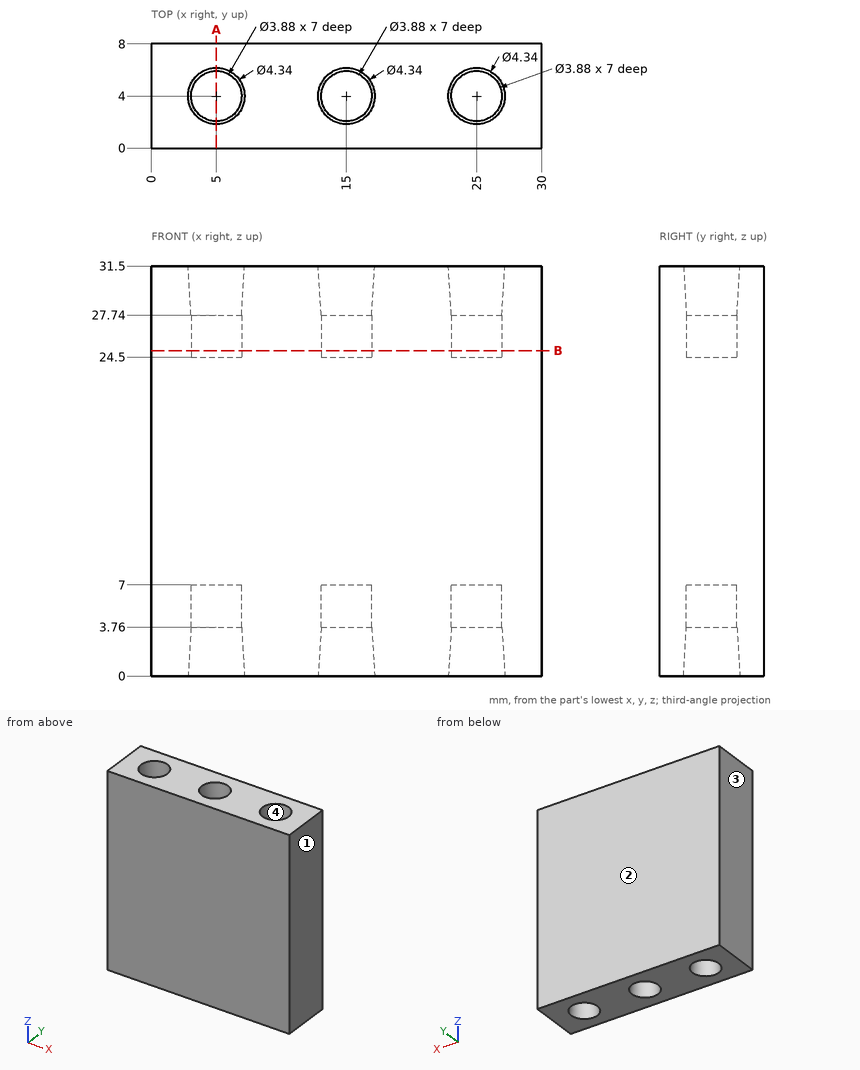
For this review, use the dimensioned drawing (mm, ordinates from the lowest corner) and the shaded views. Round coordinates to 2 decimals unless told otherwise and drop trailing zeros. Loops run counter-clockwise (first coordinate to the right, second up) from the corner with the lowest first, then second, coordinate; pieces in that order, holes last. Notation, with made-up numbers: M 14,43.5 L 58,43.5 A18 cw 58,68.5 Z; hole C -2,54 d2. An arc over 180 degrees is marked long. Answer as CSV lines item,"result".
1. Insertion check: pin 1 Ø3 at (x, y) = (15, 4) entering from +Z; pin 2 Ø1.2 at (x, y) = (4.5, 3) entering from -Z. Each pin has a flat end and moves straight along its axis. Give the tip position at first contact, or say it passes through.
Outcome:
pin 1,"stops at z = 24.5"
pin 2,"stops at z = 7"
2. To check wall thickness, follow L1, parallel to X at y = 4, z = 5.5; L2, parallel to Y at x = 25, z = 5.05; L3, parallel to Z at x = 26.25, y = 3.75. State the ranges of each line that lie inside material, in increasing order. Write a range as [from, to].
Outcome:
L1,"x = [0, 3.06], [6.94, 13.06], [16.94, 23.06], [26.94, 30]"
L2,"y = [0, 2.06], [5.94, 8]"
L3,"z = [7, 24.5]"
3. We need section B-B (z = 25). Give the boundary of the cut face in (x, y).
Outcome:
outline,"M 0,0 L 30,0 L 30,8 L 0,8 Z; hole C 5,4 d3.88; hole C 15,4 d3.88; hole C 25,4 d3.88"
4. Draft analysis for pull direction X (two halves, no side actions). For the marked faces 1, 2, 3 and 4, state which applies: pulls with the +X half, pulls with the -X half, needs draft (parallel to the pull), parting line crosses it, or undercut.
Outcome:
face 1,"pulls with the +X half"
face 2,"needs draft"
face 3,"pulls with the -X half"
face 4,"undercut"
5. We need section A-A (x = 5). Give the boundary of the cut face in (y, z).
Outcome:
outline,"M 0,0 L 1.83,0 L 2.06,3.76 L 2.06,7 L 5.94,7 L 5.94,3.76 L 6.17,0 L 8,0 L 8,31.5 L 6.17,31.5 L 5.94,27.74 L 5.94,24.5 L 2.06,24.5 L 2.06,27.74 L 1.83,31.5 L 0,31.5 Z"
